from build123d import *

# Parameters (mm, degrees)
F1_DEPTH = 38.1
F2_R     = 3.048
F4_DEPTH = 116.84


with BuildPart() as f1:
    # F0 (on Front) → F1 (new body, symmetric)
    with BuildSketch(Plane.XZ):
        Polygon((0.306206, 7.981648), (10.466206, 7.981648), (0.306206, 18.141648), align=None)
        Polygon((-54.303794, -21.495858), (62.536206, -21.495858), (62.536206, 8.984142), (10.466206, 7.981648), (0.306206, 7.981648), (0.306206, 18.141648), (-12.393794, 18.141648), (-12.393794, 7.981648), (-3.503794, 7.981648), (-3.503794, -11.335858), (-37.793794, -11.335858), (-37.793794, 8.984142), (-31.443794, 8.984142), (-31.443794, 19.144142), (-44.143794, 19.144142), (-54.303794, 8.984142), align=None)
    extrude(amount=F1_DEPTH, both=True)

    # F2
    f2_edges = [f1.edges().sort_by_distance(p)[0] for p in [
        (5.386206, -38.1, 13.061648),
        (36.501206, -38.1, 8.482895),
        (62.536206, -38.1, -6.255858),
        (62.536206, 0, 8.984142),
        (10.466206, 0, 7.981648),
        (36.501206, 38.1, 8.482895),
        (5.386206, 38.1, 13.061648),
    ]]
    fillet(f2_edges, radius=F2_R)

    # F3 (on face) → F4 (cut)
    with BuildSketch(Plane.YZ.offset(62.536206)):
        Polygon((0, -11.335858), (0, -21.495858), (19.05, -21.495858), (24.915879, -11.335858), align=None)
        Polygon((-19.05, -21.495858), (0, -21.495858), (0, -11.335858), (-25.161097, -11.335858), (-21.809316, -16.716583), align=None)
    extrude(amount=-F4_DEPTH, mode=Mode.SUBTRACT)


solid = f1.part
Read the model definition and answer for the solid it produces. Units are mm, in the model's axes. A direction names the side the tool comes from. Give positions to 0.01 mm unless a question says otherwise; leave off trailing zeros. Write each loop counter-clockwise with the first axis right and the second up, starting at its lowest first coordinate (ties: lowest second). Pieces come first, ordered by that corner, then holes. Notation, with made-up numbers: (-34, 9) - (17, 9) arc R24 ccw to (17, 26) - close; hole circle Ø4 at (-32, 86.5). An arc over 180 degrees is marked (long way). Answer in a Markdown table with one row per item. Add a question column.
Item 1: Section D-D, the plane x = -22.5 is taken. Write down the section's boundary in (y, z), and give its area (3 significant figures).
Item 2: Determine the mould class of faces 6 (the face through (-37.794, -1, -1)), 7 (the face through (4.42, 37.18, 12.8)), 8 (the face through (30, 0, -11.336)), 9 (the face through (4.9, -23.5, -14)) for opening direction Y: pulls with the +Y half, pulls with the -Y half, needs draft (parallel to the pull), parting line crosses it, or undercut.
Item 3: A tool of negligible diameter and unlimited length cuts with its end or side. For faces 1 (the face through (-6, -1, 18.142)), 2 (the face through (10.549, 0.491, 8.233)), 3 (the face through (-20, 31, -11.336)), 4 (the face through (4.93, -20.45, -19.07)), 5 (the face through (3, -29, -21.496)), from which of +Z, -Z, +X, -X, +Y, -Y can it reach the whole face along a straight path? Write none if from no direction.
Item 4: Section B-B, the plane x = -35 is taken. Write down the section's boundary in (y, z), and give its area (3 significant figures).
Item 5: Flat-ended cylindrical pins translate along their axes: P1, Ø6.5, axis at x = -17.5, y = -29.5, coming from the +Z side; P2, Ø4, axis at x = -1.5, y = -11, coming from the +Z side; P3, Ø5, axis at y = 9.5, z = 12.5, coming from the -X side; P4, Ø12, axis at x = -12, z = 1.5, coming from the -Y side. Find the tip coordinate at first contact, or state that the pin passes through.
Item 6: Section C-C, the plane y = -3.5 is taken. Write down the section's boundary in (x, z), and give its area (3 significant figures).
Item 7: Find the intervals of material crossed by L1, parallel to X at y = 22, z = 4.5; L2, parallel to Z at x = -2.5, y = -13; L3, parallel to Y at x = -42.5, z = -15, in increasing order.
Item 8: Section A-A, the plane z = 2.5 is taken. Write down the section's boundary in (x, y), and give its area (3 significant figures).
Recorded:
| question | item | result |
|---|---|---|
| 1 | outline | (-38.1, -21.5) - (-19.05, -21.5) - (-21.81, -16.72) - (-25.16, -11.34) - (-38.1, -11.34) - close; (19.05, -21.5) - (38.1, -21.5) - (38.1, -11.34) - (24.92, -11.34) - close |
| 1 | area | 327 mm2 |
| 2 | face 6 | needs draft |
| 2 | face 7 | pulls with the +Y half |
| 2 | face 8 | undercut |
| 2 | face 9 | undercut |
| 3 | face 1 | +Z, +X, +Y, -Y |
| 3 | face 2 | +Z, +Y, -Y |
| 3 | face 3 | +Y, -Y |
| 3 | face 4 | +X, -X |
| 3 | face 5 | -Z, +X, -X, +Y, -Y |
| 4 | outline | (-38.1, -21.5) - (-19.05, -21.5) - (-21.81, -16.72) - (-25.16, -11.34) - (-38.1, -11.34) - close; (-38.1, 8.98) - (38.1, 8.98) - (38.1, 19.14) - (-38.1, 19.14) - close; (19.05, -21.5) - (38.1, -21.5) - (38.1, -11.34) - (24.92, -11.34) - close |
| 4 | area | 1,100 mm2 |
| 5 | P1 | stops at z = -11.34 |
| 5 | P2 | stops at z = 18.14 |
| 5 | P3 | stops at x = -53.29 |
| 5 | P4 | passes through |
| 6 | outline | (-54.3, -11.34) - (-37.79, -11.34) - (-37.79, 8.98) - (-31.44, 8.98) - (-31.44, 19.14) - (-44.14, 19.14) - (-54.3, 8.98) - close; (-12.39, 7.98) - (-3.5, 7.98) - (-3.5, -11.34) - (62.54, -11.34) - (62.54, 5.88) arc R3.05 ccw to (59.43, 8.92) - (11.76, 8.01) arc R3.05 cw to (9.55, 8.9) - (0.31, 18.14) - (-12.39, 18.14) - close |
| 6 | area | 2,000 mm2 |
| 7 | L1 | x = -54.3 to -37.79, -3.5 to 62.54 |
| 7 | L2 | z = -11.34 to 18.14 |
| 7 | L3 | y = -38.1 to -22.88, 22.8 to 38.1 |
| 8 | outline | (-54.3, -38.1) - (-37.79, -38.1) - (-37.79, 38.1) - (-54.3, 38.1) - close; (-3.5, -38.1) - (59.49, -38.1) arc R3.05 ccw to (62.54, -35.05) - (62.54, 38.1) - (-3.5, 38.1) - close |
| 8 | area | 6,290 mm2 |
